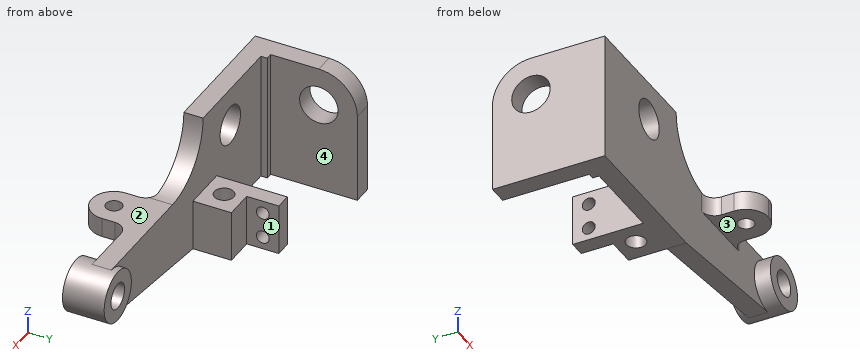
```python
from build123d import *

# Parameters (mm, degrees)
CROQUIS1_R              = 9.525
SALIENTE_EXTRUIR1_DEPTH = 9.525
CROQUIS2_W              = 9.525
CROQUIS2_H              = 63.5
SALIENTE_EXTRUIR3_DEPTH = 46.0375
CROQUIS3_R              = 9.525
CORTAR_EXTRUIR1_DEPTH   = 46.0375
CROQUIS4_R              = 12.7
SALIENTE_EXTRUIR4_DEPTH = 3.175
CROQUIS5_W              = 22.225
CROQUIS5_H              = 25.233673581
SALIENTE_EXTRUIR5_DEPTH = 19.05
CROQUIS6_W              = 7.9375
CROQUIS6_H              = 25.233673581
SALIENTE_EXTRUIR6_DEPTH = 15.875
CROQUIS7_R              = 3.175
CORTAR_EXTRUIR2_DEPTH   = 15.875
CROQUIS8_R              = 4.7625
CORTAR_EXTRUIR4_DEPTH   = 26.233673581
CROQUIS9_R              = 12.7
SALIENTE_EXTRUIR7_DEPTH = 7.9375
CROQUIS10_R             = 6.35
CORTAR_EXTRUIR5_DEPTH   = 21.6375
CROQUIS14_W             = 22.225
CROQUIS14_H             = 9.525
SALIENTE_EXTRUIR8_DEPTH = 23.8125
CROQUIS15_R             = 3.96875
CORTAR_EXTRUIR7_DEPTH   = 35.925
REDONDEO6_R             = 6.35
CROQUIS16_W             = 3.175
CROQUIS16_H             = 3.175
SALIENTE_EXTRUIR9_DEPTH = 63.5


with BuildPart() as part:
    # Croquis1 → Saliente-Extruir1 (new body)
    with BuildSketch(Plane(origin=(0, 0, 0), x_dir=(1, 0, 0), z_dir=(0, 1, 0))):
        with BuildLine():
            Line((0, 0), (66.675, 0))
            ThreePointArc((66.675, 0), (75.044423728, 20.205576272), (95.25, 28.575))
            Line((95.25, 28.575), (152.4, 28.575))
            ThreePointArc((152.4, 28.575), (165.1, 41.275), (152.4, 53.975))
            Line((152.4, 53.975), (76.2, 63.5))
            Line((76.2, 63.5), (61.9125, 63.5))
            Line((61.9125, 63.5), (9.525, 63.5))
            Line((9.525, 63.5), (0, 63.5))
            Line((0, 63.5), (0, 0))
        make_face()
        with Locations((41.275, 19.05)):
            Circle(CROQUIS1_R, mode=Mode.SUBTRACT)
    extrude(amount=SALIENTE_EXTRUIR1_DEPTH)

    # Croquis2 → Saliente-Extruir3 (add)
    with BuildSketch(Plane(origin=(0, 9.525, 0), x_dir=(1, 0, 0), z_dir=(0, 1, 0))):
        with Locations((4.7625, 31.75)):
            Rectangle(CROQUIS2_W, CROQUIS2_H)
    extrude(amount=SALIENTE_EXTRUIR3_DEPTH)

    # Croquis3 → Cortar-Extruir1 (cut)
    with BuildSketch(Plane(origin=(9.525, 0, 0), x_dir=(0, 0, -1), z_dir=(1, 0, 0))):
        with Locations((19.05, 36.5125)):
            Circle(CROQUIS3_R)
        with BuildLine():
            Line((0, 55.5625), (0, 36.5125))
            ThreePointArc((0, 36.5125), (5.579615818, 49.982884182), (19.05, 55.5625))
            Line((19.05, 55.5625), (0, 55.5625))
        make_face()
    extrude(amount=-CORTAR_EXTRUIR1_DEPTH, mode=Mode.SUBTRACT)

    # Croquis4 → Saliente-Extruir4 (add)
    with BuildSketch(Plane(origin=(0, 9.525, 0), x_dir=(1, 0, 0), z_dir=(0, 1, 0))):
        with Locations((152.4, 41.275)):
            Circle(CROQUIS4_R)
    extrude(amount=SALIENTE_EXTRUIR4_DEPTH)

    # Croquis5 → Saliente-Extruir5 (add)
    with BuildSketch(Plane(origin=(0, 9.525, 0), x_dir=(1, 0, 0), z_dir=(0, 1, 0))):
        with Locations((65.0875, 50.88316321)):
            Rectangle(CROQUIS5_W, CROQUIS5_H)
    extrude(amount=SALIENTE_EXTRUIR5_DEPTH)

    # Croquis6 → Saliente-Extruir6 (add)
    with BuildSketch(Plane(origin=(0, 28.575, 0), x_dir=(1, 0, 0), z_dir=(0, 1, 0))):
        with Locations((57.94375, 50.88316321)):
            Rectangle(CROQUIS6_W, CROQUIS6_H)
    extrude(amount=SALIENTE_EXTRUIR6_DEPTH)

    # Croquis7 → Cortar-Extruir2 (cut)
    with BuildSketch(Plane(origin=(61.9125, 0, 0), x_dir=(0, 0, -1), z_dir=(1, 0, 0))):
        with Locations((44.616326419, 36.5125)):
            Circle(CROQUIS7_R)
        with Locations((57.316326419, 36.5125)):
            Circle(CROQUIS7_R)
    extrude(amount=-CORTAR_EXTRUIR2_DEPTH, mode=Mode.SUBTRACT)

    # Croquis8 → Cortar-Extruir4 (cut, through all)
    with BuildSketch(Plane.XY.offset(-38.266326419)):
        with Locations((65.0875, 19.05)):
            Circle(CROQUIS8_R)
    extrude(amount=-CORTAR_EXTRUIR4_DEPTH, mode=Mode.SUBTRACT)

    # Croquis9 → Saliente-Extruir7 (add)
    with BuildSketch(Plane.XZ):
        with Locations((152.4, -41.275)):
            Circle(CROQUIS9_R)
    extrude(amount=SALIENTE_EXTRUIR7_DEPTH)

    # Croquis10 → Cortar-Extruir5 (cut, through all)
    with BuildSketch(Plane(origin=(0, 12.7, 0), x_dir=(1, 0, 0), z_dir=(0, 1, 0))):
        with Locations((152.4, 41.275)):
            Circle(CROQUIS10_R)
    extrude(amount=-CORTAR_EXTRUIR5_DEPTH, mode=Mode.SUBTRACT)

    # Croquis14 → Saliente-Extruir8 (add)
    with BuildSketch(Plane.XZ):
        with Locations((107.95, -33.3375)):
            Rectangle(CROQUIS14_W, CROQUIS14_H)
    extrude(amount=SALIENTE_EXTRUIR8_DEPTH)

    # Croquis15 → Cortar-Extruir7 (cut, through all)
    with BuildSketch(Plane.XY.offset(-28.575)):
        with Locations((107.95, -12.7)):
            Circle(CROQUIS15_R)
        with BuildLine():
            ThreePointArc((119.0625, -12.7), (115.807724106, -20.557724106), (107.95, -23.8125))
            Line((107.95, -23.8125), (119.0625, -23.8125))
            Line((119.0625, -23.8125), (119.0625, -12.7))
        make_face()
        with BuildLine():
            ThreePointArc((107.95, -23.8125), (100.092275894, -20.557724106), (96.8375, -12.7))
            Line((96.8375, -12.7), (96.8375, -23.8125))
            Line((96.8375, -23.8125), (107.95, -23.8125))
        make_face()
    extrude(amount=-CORTAR_EXTRUIR7_DEPTH, mode=Mode.SUBTRACT)

    # Redondeo6
    redondeo6_edges = [part.edges().sort_by_distance(p)[0] for p in [
        (119.0625, 0, -33.3375),
        (96.8375, 0, -33.3375),
    ]]
    fillet(redondeo6_edges, radius=REDONDEO6_R)

    # Croquis16 → Saliente-Extruir9 (add)
    with BuildSketch(Plane.XY):
        with Locations((11.1125, 11.1125)):
            Rectangle(CROQUIS16_W, CROQUIS16_H)
    extrude(amount=-SALIENTE_EXTRUIR9_DEPTH)


solid = part.part
```
The listing builds one solid part. Answer for the finished solid, in the listing's coordinates (mm). Face numbers are marked on the shaded views. A direction names the side the tool comes from. Give positions to 0.01 mm unless a question says otherwise; leave off trailing zeros. Order: outer loops, then holes, each group sorted by start corner. A loop starts at its lowest first (then second) coordinate and runs counter-clockwise, first axis right, second up.
Item 1: The part is cut by section D-D, the plane x = 24. Give the vertices of the cut face in (y, z) (3 decimals), and give its area (3 significant figures).
From the geometry:
outline: (0, -63.5) - (9.525, -63.5) - (9.525, 0) - (0, 0) - close
area: 605 mm2
Item 2: Which of the six approach directions +Z, -Z, +X, -X, +Y, -Y give full straight-line access (tool end or side, diameter ignored) to the marked faces 1, 2, 3 and 4?
From the geometry:
face 1: +Z, -Z, +X, +Y
face 2: +Z, +X, +Y, -Y
face 3: -Z, -X, -Y
face 4: +Z, -Z, +Y
Item 3: Find the intervals of material crossed by probe 1 along X at (y, z) = (36.5, -38.5) (1 decimal); probe 2 along Y at (x, z) = (107.95, -34.5) (1 decimal); probe 3 along Z at (x, y) = (152.4, -0.25) (3 decimals), in increasing order.
From the geometry:
probe 1: x = 0 to 9.5, 54 to 61.9
probe 2: y = -23.8 to -16.7, -8.7 to 9.5
probe 3: z = -53.975 to -47.625, -34.925 to -28.575
Item 4: The part is cut by section C-C, the plane y = -15. Give the vertices of the cut face in (x, z) (3 decimals).
From the geometry:
outline: (97.078, -38.1) - (104.716, -38.1) - (104.716, -28.575) - (97.078, -28.575) - close; (111.184, -38.1) - (118.822, -38.1) - (118.822, -28.575) - (111.184, -28.575) - close
Item 5: The part is cut by section A-A, the plane y = 19.05. Give the vertices of the cut face in (x, z) (3 decimals), and give its area (3 significant figures).
From the geometry:
outline: (0, -63.5) - (9.525, -63.5) - (9.525, 0) - (0, 0) - close; (53.975, -63.5) - (60.325, -63.5) - (60.325, -38.266) - (53.975, -38.266) - close; (69.85, -63.5) - (76.2, -63.5) - (76.2, -38.266) - (69.85, -38.266) - close
area: 925 mm2
Item 6: Given pin 1 Ø5 at (y, z) = (-10.5, -32) entering from -X; pin 2 Ø1.6 at (x, z) = (11.5, -40) entering from +Y; pin 3 Ø6 at (x, z) = (54, -29) entering from -Y; pin 4 Ø12 at (x, y) = (84.5, 20.5) entering from +Z, each flat-ended and moving along its own axis, determine where each tip first touches the part or whether it passes through.
From the geometry:
pin 1: stops at x = 96.84
pin 2: stops at y = 12.7
pin 3: stops at y = 0
pin 4: passes through
